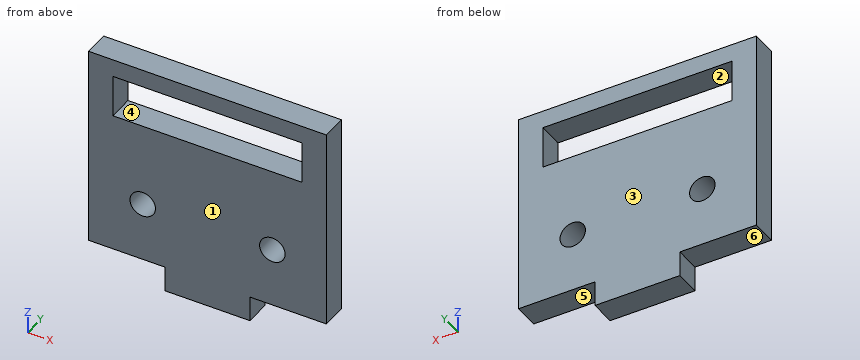
```python
from build123d import *

# Parameters (mm, degrees)
SKETCH1_R           = 1.5
SKETCH1_W           = 22.26
SKETCH1_H           = 5
BOSS_EXTRUDE1_DEPTH = 3


with BuildPart() as part:
    # Sketch1 → Boss-Extrude1 (new body)
    with BuildSketch(Plane(origin=(0, 0, 0), x_dir=(1, 0, 0), z_dir=(0, 1, 0))):
        Polygon((-5, 3), (5, 3), (14, 3), (14, 27), (5, 27), (5, 30), (-5, 30), (-5, 27), (-14, 27), (-14, 3), align=None)
        with Locations(Location((7.63, 20, 0), (0, 0, 270))):
            Circle(SKETCH1_R, mode=Mode.SUBTRACT)
        with Locations(Location((-7.63, 20, 0), (0, 0, 90))):
            Circle(SKETCH1_R, mode=Mode.SUBTRACT)
        with Locations((0, 7.6)):
            Rectangle(SKETCH1_W, SKETCH1_H, mode=Mode.SUBTRACT)
    extrude(amount=BOSS_EXTRUDE1_DEPTH)


solid = part.part
```
Could you check a few things on this model? Use its own coordinates, in mm. Face numbers are marked on the shaded views. A direction names the side the tool comes from. Give positions to 0.01 mm unless a question says otherwise; leave off trailing zeros. Loops run counter-clockwise (first coordinate to the right, second up) from the corner with the lowest first, then second, coordinate; pieces in that order, holes last. Notation, with made-up numbers: (-39.5, 54) - (-3.5, 54) arc R5 cw to (-3.5, 58) - close; hole circle Ø5 at (-16, 35). An arc over 180 degrees is marked (long way). Answer in a Markdown table with one row per item. Add a question column.
Q1. For pin 1 (0.9 mm diameter, centred on x = 11.5, y = 2, fed in from -Z), with a flat end and sliding along its axis, tell me the tip position at first contact or that it passes through.
Q2. Please list where these lines run through material, in increasing order: L1, parallel to X at y = 1.2, z = -20; L2, parallel to Z at x = -7.63, y = 0.85; L3, parallel to X at y = 2.05, z = -8. Write a range as from..to.
Q3. If we section it at C-C (x = -5.5): List the corners of the cut face in (y, z) for me, plus the area to 3 significant figures.
Q4. If we section it at D-D (x = 7.63): List the corners of the cut face in (y, z) for me, plus the area to 3 significant figures.
Q5. We'd pull the mould along X, two halves only. Please class the marked faces 1 and 2: +X half, -X half, draft (parallel to the pull), parting line (faces both ways), or undercut.
Q6. If we section it at B-B (y = 1.7): List the corners of the cut face in (x, z) for me, plus the area to 3 significant figures.
Q7. Which directions (+Z, -Z, +X, -X, +Y, -Y) give clear straight access to the entire face, cutting with the end or side of a thin tool? Please do the marked faces 3, 4, 5 and 6.
Q8. If we section it at A-A (z = -20): List the corners of the cut face in (x, y) for me, plus the area to 3 significant figures.
The answers:
| question | item | result |
|---|---|---|
| 1 | pin 1 | stops at z = -27 |
| 2 | L1 | x = -14..-9.13, -6.13..6.13, 9.13..14 |
| 2 | L2 | z = -27..-21.5, -18.5..-10.1, -5.1..-3 |
| 2 | L3 | x = -14..-11.13, 11.13..14 |
| 3 | outline | (0, -27) - (3, -27) - (3, -10.1) - (0, -10.1) - close; (0, -5.1) - (3, -5.1) - (3, -3) - (0, -3) - close |
| 3 | area | 57.0 mm^2 |
| 4 | outline | (0, -27) - (3, -27) - (3, -21.5) - (0, -21.5) - close; (0, -18.5) - (3, -18.5) - (3, -10.1) - (0, -10.1) - close; (0, -5.1) - (3, -5.1) - (3, -3) - (0, -3) - close |
| 4 | area | 48.0 mm^2 |
| 5 | face 1 | draft |
| 5 | face 2 | undercut |
| 6 | outline | (-14, -27) - (-5, -27) - (-5, -30) - (5, -30) - (5, -27) - (14, -27) - (14, -3) - (-14, -3) - close; hole (-11.13, -10.1) - (11.13, -10.1) - (11.13, -5.1) - (-11.13, -5.1) - close; hole circle Ø3 at (-7.63, -20); hole circle Ø3 at (7.63, -20) |
| 6 | area | 577 mm^2 |
| 7 | face 3 | +Z, -Z, +X, -X, +Y |
| 7 | face 4 | +Y, -Y |
| 7 | face 5 | -Z, +X, +Y, -Y |
| 7 | face 6 | -Z, -X, +Y, -Y |
| 8 | outline | (-14, 0) - (-9.13, 0) - (-9.13, 3) - (-14, 3) - close; (-6.13, 0) - (6.13, 0) - (6.13, 3) - (-6.13, 3) - close; (9.13, 0) - (14, 0) - (14, 3) - (9.13, 3) - close |
| 8 | area | 66.0 mm^2 |
